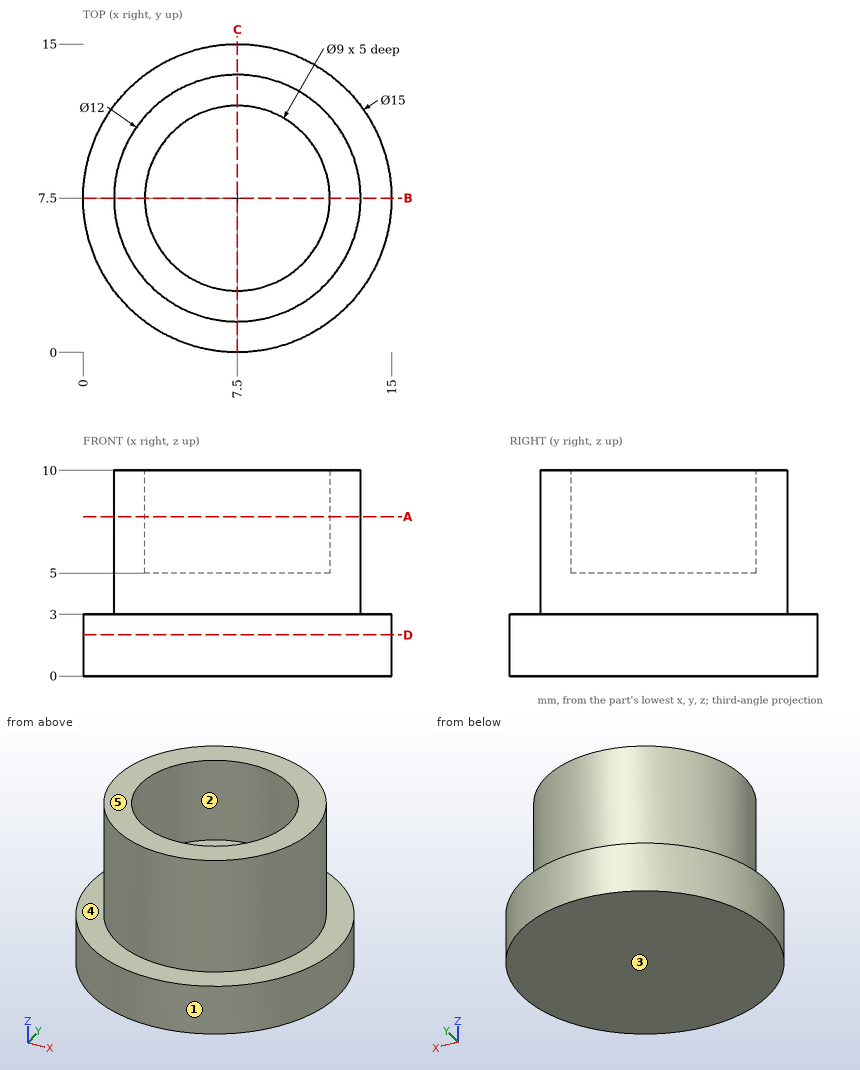
For this review, use the dimensioned drawing (mm, ordinates from the lowest corner) and the shaded views. A direction names the side the tool comes from. Coordinates: 2 decimals unless noted, no trailing zeros. Write each loop counter-clockwise with the first axis right and the second up, starting at its lowest first coordinate (ties: lowest second). Pieces come first, ordered by that corner, then holes. Notation, with made-up numbers: (69, 12.5) - (127, 12.5) arc R33 ccw to (127, 41.5) - close; hole circle Ø2 at (-29.75, 14). An arc over 180 degrees is marked (long way). One line per item, written item: value.
1) For the marked faces 4 and 5, list the 3-axis set-ups (+Z, -Z, +X, -X, +Y, -Y) from which the entire face can be reached by the end or side of a thin tool; tool diameter is ignored.
Answer sheet:
face 4: +Z
face 5: +Z, +X, -X, +Y, -Y
2) Add section A-A (z = 7.75). State the section outline as (x, y) points.
Answer sheet:
outline: circle Ø12 at (7.5, 7.5); hole circle Ø9 at (7.5, 7.5)
3) To check wall thickness, follow probe 1 along Y at (x, z) = (7.5, 7.6); probe 2 along Z at (x, y) = (3.75, 9.75); probe 3 along Z at (x, y) = (13.75, 5). State the ranges of each line that lie inside material, in increasing order.
Answer sheet:
probe 1: y = 1.5 to 3, 12 to 13.5
probe 2: z = 0 to 5
probe 3: z = 0 to 3
4) Insertion check: pin 1 (2 mm diameter, centred on y = 12.5, z = 3.5, fed in from -X); pin 2 (6 mm diameter, centred on x = 6.5, z = 7.5, fed in from -Y); pin 3 (5 mm diameter, centred on y = 2, z = 2.5, fed in from +X). Each pin has a flat end and moves straight along its axis. Give the tip position at first contact, or say it passes through.
Answer sheet:
pin 1: stops at x = 1.24
pin 2: stops at y = 1.5
pin 3: stops at x = 14.37
5) Add section B-B (y = 7.5). State the section outline as (x, z) points.
Answer sheet:
outline: (0, 0) - (15, 0) - (15, 3) - (13.5, 3) - (13.5, 10) - (12, 10) - (12, 5) - (3, 5) - (3, 10) - (1.5, 10) - (1.5, 3) - (0, 3) - close
6) Mouldability with a two-part tool opening along Y and no side actions: class the marked faces 1, 2 and 3 as +Y half, -Y half, draft (parallel to the pull), parting line (faces both ways), or undercut.
Answer sheet:
face 1: parting line
face 2: undercut
face 3: draft
7) Add section D-D (z = 2). State the section outline as (x, y) points, plus the area to 3 significant figures.
Answer sheet:
outline: circle Ø15 at (7.5, 7.5)
area: 177 mm2
